Build history of the part. All positions in model axes, mm. A direction names the side the tool comes from. Round coordinates to 2 decimals unless told otherwise and drop trailing zeros. Order: outer loops, then holes, each group sorted by start corner. A loop starts at its lowest first (then second) coordinate and runs counter-clockwise, first axis right, second up. Notation, with made-up numbers: (12, -28.75) -> (44, -28.75) arc R24 ccw to (44, -9.75) -> close; hole circle Ø4 at (-6.5, 72.5). An arc over 180 degrees is marked (long way). Answer as a JSON object with one key per item and string values.
from build123d import *

# Parameters (mm, degrees)
SKETCH1_R           = 2
BOSS_EXTRUDE1_DEPTH = 1
SKETCH2_R           = 14.5
BOSS_EXTRUDE7_DEPTH = 15.35
BOSS_EXTRUDE7_TAPER = 20
SKETCH5_R           = 7.3
CUT_EXTRUDE1_DEPTH  = 2.4


with BuildPart() as part:
    # Sketch1 → Boss-Extrude1 (new body)
    with BuildSketch(Plane.XY):
        with BuildLine():
            Line((-23.852790838, 0.920895504), (-10.258451011, 12.278606715))
            ThreePointArc((-10.258451011, 12.278606715), (0, 16), (10.258451011, 12.278606715))
            Line((10.258451011, 12.278606715), (23.852790838, 0.920895504))
            ThreePointArc((23.852790838, 0.920895504), (24.283407012, 0), (23.852790838, -0.920895504))
            Line((23.852790838, -0.920895504), (10.258451011, -12.278606715))
            ThreePointArc((10.258451011, -12.278606715), (0, -16), (-10.258451011, -12.278606715))
            Line((-10.258451011, -12.278606715), (-23.852790838, -0.920895504))
            ThreePointArc((-23.852790838, -0.920895504), (-24.283407012, 0), (-23.852790838, 0.920895504))
        make_face()
        with Locations((-19.19, 0)):
            Circle(SKETCH1_R, mode=Mode.SUBTRACT)
        with Locations(Location((19.19, 0, 0), (0, 0, 180))):
            Circle(SKETCH1_R, mode=Mode.SUBTRACT)
    extrude(amount=BOSS_EXTRUDE1_DEPTH)

    # Sketch2 → Boss-Extrude7 (add)
    with BuildSketch(Plane.XY.offset(1)):
        Circle(SKETCH2_R)
    extrude(amount=BOSS_EXTRUDE7_DEPTH, taper=BOSS_EXTRUDE7_TAPER)

    # Sketch5 → Cut-Extrude1 (cut)
    with BuildSketch(Plane.XY.offset(16.35)):
        Circle(SKETCH5_R)
    extrude(amount=-CUT_EXTRUDE1_DEPTH, mode=Mode.SUBTRACT)

    # Sketch6 → Revolve3 (revolve)
    with BuildSketch(Plane.XY.offset(13.95)):
        with BuildLine():
            Line((0, -7.3), (0, 7.3))
            ThreePointArc((0, 7.3), (-7.3, 0), (0, -7.3))
        make_face()
    revolve(axis=Axis((0, -7.3, 13.95), (0, 1, 0)))


solid = part.part
1) Probe L1, parallel to Z at x = -8, y = 0; L2, parallel to Y at x = 19.19, z = 0.2; L3, parallel to Y at x = 1, z = 5.25. List the from-to ranges inside material, lowest first. Write a range as from..to.
Checked values:
{"L1": "z = 0..16.35", "L2": "y = -4.82..-2, 2..4.82", "L3": "y = -12.91..12.91"}
2) Cut at A-A, the plane y = 0. Give the cut face in (x, z), plus the area to 3 significant figures.
Checked values:
{"outline": "(-24.28, 0) -> (-21.19, 0) -> (-21.19, 1) -> (-24.28, 1) -> close; (-17.19, 0) -> (17.19, 0) -> (17.19, 1) -> (14.5, 1) -> (8.91, 16.35) -> (7.3, 16.35) -> (7.3, 13.95) arc R7.3 ccw to (-7.3, 13.95) -> (-7.3, 16.35) -> (-8.91, 16.35) -> (-14.5, 1) -> (-17.19, 1) -> close; (21.19, 0) -> (24.28, 0) -> (24.28, 1) -> (21.19, 1) -> close", "area": "449 mm²"}
3) Cut at C-C, the plane x = 0. Give the cut face in (y, z).
Checked values:
{"outline": "(-16, 0) -> (16, 0) -> (16, 1) -> (14.5, 1) -> (8.91, 16.35) -> (7.3, 16.35) -> (7.3, 13.95) arc R7.3 ccw to (-7.3, 13.95) -> (-7.3, 16.35) -> (-8.91, 16.35) -> (-14.5, 1) -> (-16, 1) -> close"}
4) Pull direction X, two halves, no side cores. Call faces 3 (the face through (21.188, -0.088, 0.493)), 4 (the face through (-24.283, -0.015, 0.493)), 5 (the face through (0.2, -16, 0.5)): pulls with the +X half, pulls with the -X half, needs draft (parallel to the pull), parting line crosses it, or undercut.
Checked values:
{"face 3": "undercut", "face 4": "pulls with the -X half", "face 5": "parting line crosses it"}
5) Cut at D-D, the plane x = 19. Give the cut face in (y, z), plus the area to 3 significant figures.
Checked values:
{"outline": "(-4.98, 0) -> (-1.99, 0) -> (-1.99, 1) -> (-4.98, 1) -> close; (1.99, 0) -> (4.98, 0) -> (4.98, 1) -> (1.99, 1) -> close", "area": "5.97 mm²"}
6) Flat gauge pins, fed straight in: pin 1 Ø5 at (y, z) = (-4.5, 10) entering from -X; pin 2 Ø9 at (x, y) = (0.5, 0.5) entering from +Z; pin 3 Ø12 at (x, z) = (15.5, 2) entering from -Y; pin 4 Ø8 at (x, z) = (5, 14.5) entering from +Y. Where does each tip first touch, or does it go through?
Checked values:
{"pin 1": "stops at x = -11.57", "pin 2": "stops at z = 21.25", "pin 3": "stops at y = -12.81", "pin 4": "stops at y = 10.43"}
7) Cut at B-B, the plane x = -19.19. Give the cut face in (y, z).
Checked values:
{"outline": "(-4.82, 0) -> (-2, 0) -> (-2, 1) -> (-4.82, 1) -> close; (2, 0) -> (4.82, 0) -> (4.82, 1) -> (2, 1) -> close"}
8) Which spindle directions (+Z, -Z, +X, -X, +Y, -Y) get a long thin tool onto all of the face, cutting with end or side? Do faces 1 (the face through (-16.96, -6.68, 0.49)), 2 (the face through (-3, -7, 16.35)). Say none if no direction does.
Checked values:
{"face 1": "+Z, -Z, -X, -Y", "face 2": "+Z"}
